Source: CAD feature listing. Evaluate the final solid. Frame: model axes, mm. A direction names the side the tool comes from. Round coordinates to 2 decimals unless told otherwise and drop trailing zeros. Write each loop counter-clockwise with the first axis right and the second up, starting at its lowest first coordinate (ties: lowest second). Pieces come first, ordered by that corner, then holes.
Autodesk Fusion 360 part; units mm, degrees
sketch "Sketch1" plane through (0, 0, 0) normal (0, 1, 0) x (1, 0, 0)
  line L0 (50, 25) -> (-50, 25)
  line L1 (-50, 25) -> (-50, -25)
  line L2 (-50, -25) -> (50, -25)
  line L3 (50, -25) -> (50, 25)
  line L4 (50, 25) -> (-50, -25) construction
  line L5 (-50, 25) -> (50, -25) construction
  line L6 (0, 0) -> (0, 15) construction
  line L7 (0, 0) -> (-17.4892, 0) construction
  circle A0 centre (42.83, 6.35) radius 1.75
  circle A1 centre (-30, 6.35) radius 1.75
  circle A2 centre (-9.85, -13.8) radius 1.75
  line L8 (70, 7.5) -> (50, 7.5)
  line L9 (50, 7.5) -> (50, -7.5)
  line L10 (50, -7.5) -> (70, -7.5)
  line L11 (70, -7.5) -> (70, 7.5)
  line L12 (70, 7.5) -> (50, -7.5) construction
  line L13 (50, 7.5) -> (70, -7.5) construction
  line L14 (-70, 7.5) -> (-50, 7.5)
  line L15 (-70, -7.5) -> (-70, 7.5)
  line L16 (-50, -7.5) -> (-70, -7.5)
  circle A3 centre (62, 0) radius 3.4
  circle A4 centre (-62, 0) radius 3.4
  line L17 (42.83, 6.35) -> (-30, 6.35) construction
  point P0 (60, 0)
  dimension "d1" = 3.5
  dimension "d2" = 3.5
  dimension "d3" = 3.5
  dimension "d4" = 6.8
  dimension "d5" = 15
  dimension "d6" = 20
  dimension "d7" = 12
  dimension "d8" = 100
  dimension "d9" = 50
  dimension "d10" = 72.83
  dimension "d11" = 20.15
  dimension "d12" = 20.15
  dimension "d13" = 20
  dimension "d14" = 18.65
extrude "Extrude1" add sketch "Sketch1" along normal blind 4
fillet "Fillet1" radius 3 12 edges at (50, 2, 7.5) (50, 2, 25) (70, 2, 7.5) (70, 2, -7.5) (50, 2, -7.5) (50, 2, -25) (-50, 2, -25) (-50, 2, -7.5) (-70, 2, -7.5) (-70, 2, 7.5) (-50, 2, 7.5) (-50, 2, 25)
chamfer "Chamfer1" distance 2 angle 45 3 edges at (41.1984, 4, -6.9828) (-11.4816, 4, 13.1672) (-31.6316, 4, -6.9828)
1) Reachability of faces 4 (the face through (50, 2, -16)), 5 (the face through (60, 2, 7.5)), 6 (the face through (-50, 2, -16)), 7 (the face through (-50, 2, 16)) from +Z, -Z, +X, -X, +Y, -Y: full face, straight path, thin tool, end or side. Return the list, or none.
Taken from the geometry:
face 4: -Z, +X, +Y, -Y
face 5: +Z, +X, +Y, -Y
face 6: -Z, -X, +Y, -Y
face 7: +Z, -X, +Y, -Y
2) Section query A-A on x = -30. Return the cut outline in (y, z).
Taken from the geometry:
outline: (0, -25) - (4, -25) - (4, -10.1) - (2, -8.1) - (0, -8.1) - close; (0, -4.6) - (2, -4.6) - (4, -2.6) - (4, 25) - (0, 25) - close
3) Section query D-D on x = -62. Return the cut outline in (y, z), then the cut area to 3 significant figures.
Taken from the geometry:
outline: (0, -7.5) - (4, -7.5) - (4, -3.4) - (0, -3.4) - close; (0, 3.4) - (4, 3.4) - (4, 7.5) - (0, 7.5) - close
area: 32.8 mm2
4) Pull-direction query (X, two-part tool) for faces 1 (the face through (60, 2, -7.5)), 2 (the face through (70, 2, 0)), 3 (the face through (-10.256, 2.125, 15.631)); classes: released by +X, released by -X, zero draft, split by the parting line, or undercut.
Taken from the geometry:
face 1: zero draft
face 2: released by +X
face 3: undercut
5) Section query B-B on z = 13.8. Return the cut outline in (x, y), then the cut area to 3 significant figures.
Taken from the geometry:
outline: (-50, 0) - (-11.6, 0) - (-11.6, 2) - (-13.6, 4) - (-50, 4) - close; (-8.1, 0) - (50, 0) - (50, 4) - (-6.1, 4) - (-8.1, 2) - close
area: 382 mm2
6) Contact query for flat-ended pins moving along their axis: P1, Ø2, axis at x = 59.5, y = 2.5, coming from the +Z side; P2, Ø2, axis at y = 1, z = 17, coming from the +X side; P3, Ø1.2, axis at y = 1, z = -15, coming from the -X side. Output: stop coordinate, or through.
Taken from the geometry:
P1: stops at z = 7.5
P2: stops at x = 50
P3: stops at x = -50
7) Section query C-C on y = 1.15. State how many separate pieces and enclosed holes the cut face has, then the cut area to 3 significant figures.
Taken from the geometry:
separate pieces: 1
enclosed holes: 5
area: 5,490 mm2
8) Material intervals for line 1 (X direction, y = 1.6, z = 0); line 2 (X direction, y = 1.5, z = -6.35); line 3 (Z direction, x = -62, y = 1.5), sorted ascending.
Taken from the geometry:
line 1: x = -70 to -65.4, -58.6 to 58.6, 65.4 to 70
line 2: x = -69.36 to -31.75, -28.25 to 41.08, 44.58 to 69.36
line 3: z = -7.5 to -3.4, 3.4 to 7.5
